```python
from build123d import *

# Parameters (mm, degrees)
F0_W     = 4
F0_H     = 24.11321
F0_W_2   = 22.79535
F0_H_2   = 4
F0_W_3   = 17.79535
F1_DEPTH = 30
F2_R     = 1.5
F3_DEPTH = 25
F4_R     = 1.5
F5_DEPTH = 25


with BuildPart() as f1:
    # F0 (on Right) → F1 (new body)
    with BuildSketch(Plane.YZ):
        with Locations((-14.226417, 12.056605)):
            Rectangle(F0_W, F0_H)
        with Locations((8.171258, 7)):
            Rectangle(F0_W_2, F0_H_2)
        with Locations((10.671258, -2)):
            Rectangle(F0_W_3, F0_H_2)
        Polygon((1.773583, -4), (1.773583, 0), (-3.226417, 0), (-7.226417, 0), (-12.226417, 0), (-16.226417, 0), (-16.226417, -4), align=None)
        Polygon((-7.226417, 0), (-3.226417, 0), (-3.226417, 5), (-3.226417, 9), (-3.226417, 24.11321), (-7.226417, 24.11321), align=None)
    extrude(amount=F1_DEPTH)

    # F2 (on face) → F3 (cut)
    with BuildSketch(Plane(origin=(0, -3.226417, 0), x_dir=(-1, 0, 0), z_dir=(0, 1, 0))):
        with Locations((-18.920988, 18.018588)):
            Circle(F2_R)
        with Locations((-7.910667, 16.17527)):
            Circle(F2_R)
    extrude(amount=-F3_DEPTH, mode=Mode.SUBTRACT)

    # F4 (on face) → F5 (cut)
    with BuildSketch(Plane.XY.offset(9)):
        with Locations((8.8035, 11.279188)):
            Circle(F4_R)
        with Locations((17.396833, 11.026443)):
            Circle(F4_R)
    extrude(amount=-F5_DEPTH, mode=Mode.SUBTRACT)


solid = f1.part
```
Could you check a few things on this model? Use its own coordinates, in mm. A direction names the side the tool comes from. Coordinates: 2 decimals unless noted, no trailing zeros. Write each loop counter-clockwise with the first axis right and the second up, starting at its lowest first coordinate (ties: lowest second). Pieces come first, ordered by that corner, then holes. Notation, with made-up numbers: (-12.5, 85) -> (28.5, 85) arc R24 cw to (28.5, 116) -> close; hole circle Ø7 at (60, 69). An arc over 180 degrees is marked (long way). Return JSON: item names as keys, results as strings.
(1) Imagine slicing it at D-D, the plane z = 17. Please give me the cut outline in (x, y), then the cut area to 3 significant figures.
Numbers:
{"outline": "(0, -16.23) -> (6.66, -16.23) -> (6.66, -12.23) -> (0, -12.23) -> close; (0, -7.23) -> (6.66, -7.23) -> (6.66, -3.23) -> (0, -3.23) -> close; (9.16, -16.23) -> (17.82, -16.23) -> (17.82, -12.23) -> (9.16, -12.23) -> close; (9.16, -7.23) -> (17.82, -7.23) -> (17.82, -3.23) -> (9.16, -3.23) -> close; (20.02, -16.23) -> (30, -16.23) -> (30, -12.23) -> (20.02, -12.23) -> close; (20.02, -7.23) -> (30, -7.23) -> (30, -3.23) -> (20.02, -3.23) -> close", "area": "202 mm2"}
(2) I need wall thicknesses on L1, parallel to Z at x = 17.25, y = 18.5; L2, parallel to Y at x = 25, z = 14; L3, parallel to Y at x = 11, z = 7.75. Which ranges of each line are inside material? Lowest first, please.
Numbers:
{"L1": "z = -4 to 0, 5 to 9", "L2": "y = -16.23 to -12.23, -7.23 to -3.23", "L3": "y = -16.23 to -12.23, -7.23 to 19.57"}
(3) Which directions (+Z, -Z, +X, -X, +Y, -Y) give clear straight access to the entire face, cutting with the end or side of a thin tool? Please do faces 4 (the flat face through (15, -10, 0)), 5 (the cylindrical face through (10.189, 10.705, -1.972)), 6 (the flat face through (15, 8, 0)).
Numbers:
{"face 4": "+Z, +X, -X", "face 5": "+Z, -Z", "face 6": "+X, -X, +Y"}
(4) Imagine slicing it at A-A, the plane z = 13.5. Please give me the cut outline in (x, y), then the cut area to 3 significant figures.
Numbers:
{"outline": "(0, -16.23) -> (30, -16.23) -> (30, -12.23) -> (0, -12.23) -> close; (0, -7.23) -> (30, -7.23) -> (30, -3.23) -> (0, -3.23) -> close", "area": "240 mm2"}
(5) We'd pull the mould along Y, two halves only. Please class faces 1 (the cylindrical face through (10.189, 10.705, 7.028)), 2 (the flat face through (15, 19.569, 7)), 3 (the flat face through (30, -3, 7)): +Y half, -Y half, draft (parallel to the pull), parting line (faces both ways), or undercut.
Numbers:
{"face 1": "undercut", "face 2": "+Y half", "face 3": "draft"}
(6) I'm going to push flat-ended pins straight in: pin 1 (1.5 mm diameter, centred on x = 16.5, z = 21, fed in from +Y); pin 2 (3 mm diameter, centred on x = 24.5, y = 12.5, fed in from +Z). Where does each tip first touch, or does it pass through?
Numbers:
{"pin 1": "stops at y = -3.23", "pin 2": "stops at z = 9"}
(7) Imagine slicing it at C-C, the plane y = -0.5. Please give me the cut outline in (x, z), then the cut area to 3 significant figures.
Numbers:
{"outline": "(0, -4) -> (30, -4) -> (30, 0) -> (0, 0) -> close; (0, 5) -> (30, 5) -> (30, 9) -> (0, 9) -> close", "area": "240 mm2"}
(8) Imagine slicing it at B-B, the plane x = 19.5. Please give me the cut outline in (y, z).
Numbers:
{"outline": "(-16.23, -4) -> (19.57, -4) -> (19.57, 0) -> (-3.23, 0) -> (-3.23, 5) -> (19.57, 5) -> (19.57, 9) -> (-3.23, 9) -> (-3.23, 16.63) -> (-7.23, 16.63) -> (-7.23, 0) -> (-12.23, 0) -> (-12.23, 16.63) -> (-16.23, 16.63) -> close; (-16.23, 19.4) -> (-12.23, 19.4) -> (-12.23, 24.11) -> (-16.23, 24.11) -> close; (-7.23, 19.4) -> (-3.23, 19.4) -> (-3.23, 24.11) -> (-7.23, 24.11) -> close"}
